```python
from build123d import *

# Parameters (mm, degrees)
F0_W     = 95.25
F0_H     = 38.1
F0_R     = 2.54
F1_DEPTH = 25.4
F2_W     = 88.9
F2_H     = 20.32
F3_DEPTH = 38.101
F4_W     = 3.175
F4_H     = 19.05
F5_DEPTH = 25.4


with BuildPart() as f1:
    # F0 (on Top) → F1 (new body)
    with BuildSketch(Plane.XY):
        with Locations((47.625, 19.05)):
            Rectangle(F0_W, F0_H)
        with Locations((31.75, 19.05)):
            Circle(F0_R, mode=Mode.SUBTRACT)
        with Locations((69.85, 19.05)):
            Circle(F0_R, mode=Mode.SUBTRACT)
    extrude(amount=F1_DEPTH)

    # F2 (on face) → F3 (cut, through all)
    with BuildSketch(Plane.XZ):
        with Locations((50.8, 15.24)):
            Rectangle(F2_W, F2_H)
    extrude(amount=-F3_DEPTH, mode=Mode.SUBTRACT)

    # F4 (on face) → F5 (cut)
    with BuildSketch(Plane(origin=(0, 0, 0), x_dir=(0, -1, 0), z_dir=(-1, 0, 0))):
        with Locations((-19.05, 15.875)):
            Rectangle(F4_W, F4_H)
    extrude(amount=-F5_DEPTH, mode=Mode.SUBTRACT)


solid = f1.part
```
Source: CAD feature listing. Evaluate the final solid. Frame: model axes, mm. A direction names the side the tool comes from. Round coordinates to 2 decimals unless told otherwise and drop trailing zeros. Write each loop counter-clockwise with the first axis right and the second up, starting at its lowest first coordinate (ties: lowest second). Pieces come first, ordered by that corner, then holes. Notation, with made-up numbers: M 85.25,-24.75 L 112.25,-24.75 A6 cw 112.25,-20.75 Z; hole C 82.5,59 d2. An arc over 180 degrees is marked long. Use CSV: the item, a comma, the result in double quotes. Start each with the question number.
Q1. Cut plane D-D on y = 25.5. Output: boundary loops of the cut face in (x, z), plus the area to 3 significant figures.
Q2. First-contact query: P1, Ø6, axis at y = 13, z = 12, coming from the +X side; P2, Ø11.5, axis at x = 44, y = 15.5, coming from the +Z side; P3, Ø1.6, axis at x = 4.5, y = 19, coming from the +Z side; P4, Ø3, axis at x = 64, y = 6, coming from the -Z side. Flat tips, straight axial feed; report the tip coordinate or a pass-through.
Q3. Access query for faces 4 (the face through (3, 9, 25.4)), 5 (the face through (3, 20.638, 16)), 6 (the face through (6.35, 23, 15)). Directions: +Z, -Z, +X, -X, +Y, -Y. A direction counts if a zero-diameter tool reaches every point of the face in a straight line with its end or side. Return the directions, or none.
Q4. Pull-direction query (Y, two-part tool) for faces 1 (the face through (37, 0, 4)), 2 (the face through (72.196, 18.077, 2.504)), 3 (the face through (0, 23, 13)); classes: +Y half, -Y half, draft (parallel to the pull), parting line (faces both ways), or undercut.
Q5. Line query: line 1 (X direction, y = 19.05, z = 1.25); line 2 (Y direction, x = 69.85, z = 2.95); line 3 (X direction, y = 32.5, z = 23.75). Output: solid intervals per line, ascending. Write a range as from..to.
Q6. Cut plane B-B on z = 18.75. Output: boundary loops of the cut face in (x, y).
Q7. Cut plane C-C on x = 69.85. Output: boundary loops of the cut face in (y, z).
Q8. Cut plane A-A on y = 19.05. Output: boundary loops of the cut face in (x, z).
Results found:
1,outline,"M 0,0 L 95.25,0 L 95.25,5.08 L 6.35,5.08 L 6.35,25.4 L 0,25.4 Z"
1,area,"613 mm^2"
2,P1,"x = 6.35"
2,P2,"z = 5.08"
2,P3,"z = 6.35"
2,P4,"z = 0"
3,face 4,"+Z, +X, -X, +Y, -Y"
3,face 5,"+Z, +X, -X"
3,face 6,"+Z, +X, +Y, -Y"
4,face 1,"-Y half"
4,face 2,"undercut"
4,face 3,"draft"
5,line 1,"0..29.21, 34.29..67.31, 72.39..95.25"
5,line 2,"0..16.51, 21.59..38.1"
5,line 3,"0..6.35"
6,outline,"M 0,0 L 6.35,0 L 6.35,17.46 L 0,17.46 Z; M 0,20.64 L 6.35,20.64 L 6.35,38.1 L 0,38.1 Z"
7,outline,"M 0,0 L 16.51,0 L 16.51,5.08 L 0,5.08 Z; M 21.59,0 L 38.1,0 L 38.1,5.08 L 21.59,5.08 Z"
8,outline,"M 0,0 L 29.21,0 L 29.21,5.08 L 6.35,5.08 L 6.35,6.35 L 0,6.35 Z; M 34.29,0 L 67.31,0 L 67.31,5.08 L 34.29,5.08 Z; M 72.39,0 L 95.25,0 L 95.25,5.08 L 72.39,5.08 Z"
